Read the model definition and answer for the solid it produces. Units are mm, in the model's axes. Face numbers are marked on the shaded views. Coordinates: 2 decimals unless noted, no trailing zeros. Loops run counter-clockwise (first coordinate to the right, second up) from the corner with the lowest first, then second, coordinate; pieces in that order, holes last. Notation, with made-up numbers: (-10, 62) - (-5, 62) arc R7 cw to (-5, 69) - close; hole circle Ø2 at (-2, 35.25). An arc over 180 degrees is marked (long way). Use one line per item in the form item = value. Start each with the question number.
1) This flat-tipped pin is pushed along its axis until it touches: P1, Ø2, axis at x = -8.93, z = 19, coming from the -Y side. Where does it stop, or does it pass through?
2) A cutting plane is placed at D-D (x = -3.5). Give the vertices of the cut face in (y, z), and give its area (3 significant figures).
3) A cutting plane is placed at B-B (x = 10.5). Give the vertices of the cut face in (y, z), and give its area (3 significant figures).
4) The mould has two halves that part along X. Classify the marked faces 1, 2, 3 and 4: released by +X, released by -X, zero draft, split by the parting line, or undercut.
5) A cutting plane is placed at C-C (z = 11.5). Give the vertices of the cut face in (x, y), and give its area (3 significant figures).
6) Consider line 1 (Y direction, x = -10.5, z = 9.75); line 2 (Z direction, x = -9.5, y = 5.7); line 3 (Y direction, x = 21.5, z = 23.5). Determine where each line is inside the solid, lowest interval first.
7) A cutting plane is placed at A-A (z = 19). Give the vertices of the cut face in (x, y).
from build123d import *

# Parameters (mm, degrees)
BOSS_EXTRUDE1_DEPTH = 25
SKETCH2_R           = 1.75
CUT_EXTRUDE1_DEPTH  = 2.5
FILLET1_R           = 2


with BuildPart() as part:
    # Sketch1 → Boss-Extrude1 (new body)
    with BuildSketch(Plane.XY):
        Polygon((-19.601594954, 4.272951405), (-14.997101112, 5.948850108), (21.13187983, 5.948850108), (25.736373672, 4.272951405), (25.223343457, 2.863412474), (20.867389359, 4.448850108), (-14.732610641, 4.448850108), (-19.088564739, 2.863412474), align=None)
    extrude(amount=BOSS_EXTRUDE1_DEPTH)

    # Sketch2 → Cut-Extrude1 (cut, through all)
    with BuildSketch(Plane.XZ.offset(-4.448850108)):
        with Locations((-8.932610641, 19)):
            Circle(SKETCH2_R)
        with Locations((11.067389359, 19)):
            Circle(SKETCH2_R)
    extrude(amount=-CUT_EXTRUDE1_DEPTH, mode=Mode.SUBTRACT)

    # Fillet1
    fillet1_edges = [part.edges().sort_by_distance(p)[0] for p in [
        (-19.345079846, 3.56818194, 0),
        (25.479858564, 3.56818194, 25),
        (-19.345079846, 3.56818194, 25),
        (25.479858564, 3.56818194, 0),
    ]]
    fillet(fillet1_edges, radius=FILLET1_R)


solid = part.part
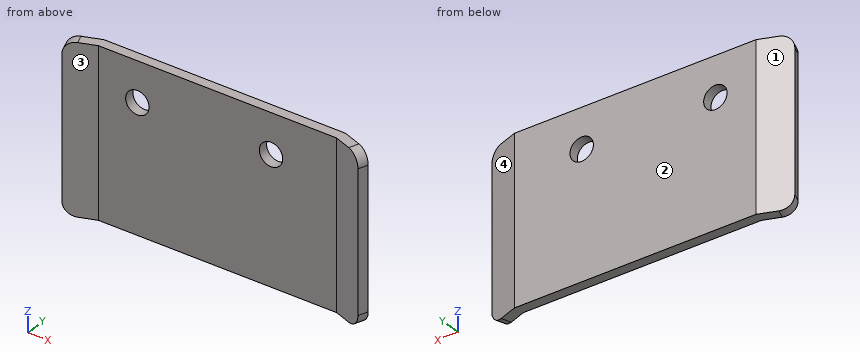
Found:
q1.P1 = through
q2.outline = (4.45, 0) - (5.95, 0) - (5.95, 25) - (4.45, 25) - close
q2.area = 37.5 mm^2
q3.outline = (4.45, 0) - (5.95, 0) - (5.95, 17.34) - (4.45, 17.34) - close; (4.45, 20.66) - (5.95, 20.66) - (5.95, 25) - (4.45, 25) - close
q3.area = 32.5 mm^2
q4.face_1 = released by -X
q4.face_2 = zero draft
q4.face_3 = undercut
q4.face_4 = released by +X
q5.outline = (-19.6, 4.27) - (-19.09, 2.86) - (-14.73, 4.45) - (20.87, 4.45) - (25.22, 2.86) - (25.74, 4.27) - (21.13, 5.95) - (-15, 5.95) - close
q5.area = 68.1 mm^2
q6.line_1 = 4.45 to 5.95
q6.line_2 = 0 to 17.34, 20.66 to 25
q6.line_3 = 4.22 to 5.81
q7.outline = (-19.6, 4.27) - (-19.09, 2.86) - (-14.73, 4.45) - (-10.68, 4.45) - (-10.68, 5.95) - (-15, 5.95) - close; (-7.18, 4.45) - (9.32, 4.45) - (9.32, 5.95) - (-7.18, 5.95) - close; (12.82, 4.45) - (20.87, 4.45) - (25.22, 2.86) - (25.74, 4.27) - (21.13, 5.95) - (12.82, 5.95) - close
